Work out the finished part from the listing and answer in its coordinate system (mm). A direction names the side the tool comes from. Give positions to 0.01 mm unless a question says otherwise; leave off trailing zeros. Order: outer loops, then holes, each group sorted by start corner. A loop starts at its lowest first (then second) coordinate and runs counter-clockwise, first axis right, second up.
```python
from build123d import *

# Parameters (mm, degrees)
EXTRUDE_1_DEPTH     = 104
SKETCH_2_R          = 2
SKETCH_2_R_2        = 2.5
SKETCH_2_R_3        = 1.5
SKETCH_2_W          = 6.5
SKETCH_2_H          = 74
CUT_EXTRUDE_1_DEPTH = 151.638640461
SKETCH_3_R          = 11.5
SKETCH_3_R_2        = 1.6
CUT_EXTRUDE_2_DEPTH = 151.638640461


with BuildPart() as part:
    # 草图1 → 凸台-拉伸1 (new body)
    with BuildSketch(Plane(origin=(0, 0, 0), x_dir=(0, 0, -1), z_dir=(1, 0, 0))):
        Polygon((0, 0), (80, 0), (80, 6), (6, 6), (6, 80), (0, 80), (0, 6), align=None)
    extrude(amount=EXTRUDE_1_DEPTH)

    # 草图2 → 切除-拉伸1 (cut, through all)
    with BuildSketch(Plane(origin=(0, 6, 0), x_dir=(1, 0, 0), z_dir=(0, 1, 0))):
        with Locations(Location((43, 11, 0), (0, 0, 270))):
            Circle(SKETCH_2_R)
        with Locations(Location((43, 35, 0), (0, 0, 270))):
            Circle(SKETCH_2_R)
        with Locations(Location((42, 48, 0), (0, 0, 270))):
            Circle(SKETCH_2_R)
        with Locations(Location((42, 72, 0), (0, 0, 270))):
            Circle(SKETCH_2_R)
        with Locations(Location((62, 72, 0), (0, 0, 90))):
            Circle(SKETCH_2_R)
        with Locations(Location((62, 48, 0), (0, 0, 90))):
            Circle(SKETCH_2_R)
        with Locations(Location((61, 35, 0), (0, 0, 90))):
            Circle(SKETCH_2_R)
        with Locations(Location((61, 11, 0), (0, 0, 90))):
            Circle(SKETCH_2_R)
        with Locations(Location((57.5, 23, 0), (0, 0, 270))):
            Circle(SKETCH_2_R_2)
        with Locations(Location((89.5, 23, 0), (0, 0, 270))):
            Circle(SKETCH_2_R_2)
        with Locations(Location((46.5, 23, 0), (0, 0, 90))):
            Circle(SKETCH_2_R_2)
        with Locations(Location((14.5, 23, 0), (0, 0, 90))):
            Circle(SKETCH_2_R_2)
        with Locations(Location((87.5, 35, 0), (0, 0, 90))):
            Circle(SKETCH_2_R_3)
        with Locations(Location((87.5, 54, 0), (0, 0, 90))):
            Circle(SKETCH_2_R_3)
        with Locations((100.75, 43)):
            Rectangle(SKETCH_2_W, SKETCH_2_H)
        with Locations((3.25, 43)):
            Rectangle(SKETCH_2_W, SKETCH_2_H)
    extrude(amount=-CUT_EXTRUDE_1_DEPTH, mode=Mode.SUBTRACT)

    # 草图3 → 切除-拉伸2 (cut, through all)
    with BuildSketch(Plane(origin=(0, 0, -6), x_dir=(-1, 0, 0), z_dir=(0, 0, -1))):
        with Locations((-52, 26)):
            Circle(SKETCH_3_R)
        with Locations((-36.5, 41.5)):
            Circle(SKETCH_3_R_2)
        with Locations(Location((-67.5, 41.5, 0), (0, 0, 180))):
            Circle(SKETCH_3_R_2)
        with Locations((-67.5, 10.5)):
            Circle(SKETCH_3_R_2)
        with Locations(Location((-36.5, 10.5, 0), (0, 0, 180))):
            Circle(SKETCH_3_R_2)
        Polygon((-97.5, 0), (-97.5, 56), (-6.5, 56), (-6.5, 0), (0, 0), (0, 80), (-104, 80), (-104, 0), align=None)
    extrude(amount=-CUT_EXTRUDE_2_DEPTH, mode=Mode.SUBTRACT)


solid = part.part
```
1. Which of the six approach directions +Z, -Z, +X, -X, +Y, -Y give full straight-line access (tool end or side, diameter ignored) to faces 4 (the face through (41, 31, -6)), 5 (the face through (40, 3, -48))?
Findings below:
face 4: -Z, +X, -X, +Y
face 5: +Y, -Y
2. The part is cut by section A-A (z = -35). Write down the section's boundary in (x, y), then the cut area to 3 significant figures.
Findings below:
outline: (6.5, 0) - (41, 0) - (41, 6) - (6.5, 6) - close; (45, 0) - (59, 0) - (59, 6) - (45, 6) - close; (63, 0) - (86, 0) - (86, 6) - (63, 6) - close; (89, 0) - (97.5, 0) - (97.5, 6) - (89, 6) - close
area: 480 mm2
3. The mould has two halves that part along X. Classify faces 1 (the face through (59, 3, -11)), 2 (the face through (53, 56, -3)), 3 (the face through (97.5, 5, -25)): pulls with the +X half, pulls with the -X half, needs draft (parallel to the pull), parting line crosses it, or undercut.
Findings below:
face 1: undercut
face 2: needs draft
face 3: pulls with the +X half
4. Given P1, Ø12, axis at x = 42, y = 31.5, coming from the -Z side; P2, Ø6, axis at x = 14.5, z = -23, coming from the +Y side, each flat-ended and moving along its own axis, determine where each tip first touches the part or whether it passes through.
Findings below:
P1: stops at z = -6
P2: stops at y = 6
5. The part is cut by section C-C (y = 17). Write down the section's boundary in (x, z).
Findings below:
outline: (6.5, -6) - (44.84, -6) - (44.84, 0) - (6.5, 0) - close; (59.16, -6) - (97.5, -6) - (97.5, 0) - (59.16, 0) - close
6. The part is cut by section D-D (z = -23). Write down the section's boundary in (x, y), then the cut area to 3 significant figures.
Findings below:
outline: (6.5, 0) - (12, 0) - (12, 6) - (6.5, 6) - close; (17, 0) - (44, 0) - (44, 6) - (17, 6) - close; (49, 0) - (55, 0) - (55, 6) - (49, 6) - close; (60, 0) - (87, 0) - (87, 6) - (60, 6) - close; (92, 0) - (97.5, 0) - (97.5, 6) - (92, 6) - close
area: 426 mm2
7. Straight lines are drawn through the part: probe 1 along X at (y, z) = (4.05, -35); probe 2 along X at (y, z) = (2, -11); probe 3 along X at (y, z) = (1.65, -23). For each, find the intervals that lie inside material, in ascending order.
Findings below:
probe 1: x = 6.5 to 41, 45 to 59, 63 to 86, 89 to 97.5
probe 2: x = 6.5 to 41, 45 to 59, 63 to 97.5
probe 3: x = 6.5 to 12, 17 to 44, 49 to 55, 60 to 87, 92 to 97.5
8. The part is cut by section B-B (x = 36.5). Write down the section's boundary in (y, z).
Findings below:
outline: (0, -80) - (6, -80) - (6, -6) - (8.9, -6) - (8.9, 0) - (0, 0) - close; (12.1, -6) - (39.9, -6) - (39.9, 0) - (12.1, 0) - close; (43.1, -6) - (56, -6) - (56, 0) - (43.1, 0) - close
